from build123d import *

# Parameters (mm, degrees)
CUT_EXTRUDE1_DEPTH      = 18.194103655
CUT_EXTRUDE1_DEPTH_BACK = 18.194103655
SKETCH3_W               = 1
SKETCH3_H               = 11


with BuildPart() as part:
    # Sketch1 → Revolve1 (revolve)
    with BuildSketch(Plane.XY, mode=Mode.PRIVATE) as revolve1_sk:
        Polygon((0, -7), (0, 0), (2.3495, 0), (2.3495, -1.27), (1.7, -1.27), (1.7, -2.92), (1.397, -2.92), (1.397, -14.77), (1.8415, -14.77), (0.889, -16.87), (0.635, -16.87), (0.635, -7), align=None)
    revolve(revolve1_sk.sketch.rotate(Axis((0, -7, 0), (0, 1, 0)), 90), axis=Axis((0, -7, 0), (0, 1, 0)))

    # Sketch3 → Cut-Extrude1 (cut, two sides: drawn at the far end of the back side and taken through both)
    with BuildSketch(Plane.XY.offset(-CUT_EXTRUDE1_DEPTH_BACK)):
        with Locations((0.029190269, -11.37)):
            Rectangle(SKETCH3_W, SKETCH3_H)
    extrude(amount=CUT_EXTRUDE1_DEPTH + CUT_EXTRUDE1_DEPTH_BACK, mode=Mode.SUBTRACT)


solid = part.part
Source: CAD feature listing. Evaluate the final solid. Frame: model axes, mm. A direction names the side the tool comes from. Coordinates: 2 decimals unless noted, no trailing zeros. Loops run counter-clockwise (first coordinate to the right, second up) from the corner with the lowest first, then second, coordinate; pieces in that order, holes last. Notation, with made-up numbers: (78.5, -18.75) -> (129.5, -18.75) arc R20 cw to (129.5, -7.75) -> close; hole circle Ø1 at (11, 79.5). An arc over 180 degrees is marked (long way). Answer in a Markdown table with one row per item. Add a question column.
Q1. Ray query, line 1 along X through (y, z) = (-10, -0.85); line 2 along X through (y, z) = (-11.25, 1.05); line 3 along Y through (x, z) = (1.5, 0.2). Return the intervals inside material, ascending.
Q2. Pull-direction query (X, two-part tool) for faces 1 (the face through (1.24, -8.93, -0.64)), 2 (the face through (0, -5.87, 0)), 3 (the face through (-1.36, -15.83, -0.02)), 4 (the face through (-0.471, -11, 1)); classes: pulls with the +X half, pulls with the -X half, needs draft (parallel to the pull), parting line crosses it, or undercut.
Q3. Reachability of faces 5 (the face through (0.529, -11, 1)), 6 (the face through (-2, -1.27, 0)), 7 (the face through (-1.6, -14.77, 0)) from +Z, -Z, +X, -X, +Y, -Y: full face, straight path, thin tool, end or side. Return the list, or none.
Q4. Section C-C on y = -13. Return the cut outline in (x, z) (3 decimals), and give its area (3 significant figures).
Q5. Section A-A on x = 0. Return the cut outline in (y, z).
Q6. Contact query for flat-ended pins moving along their axis: pin 1 Ø0.7 at (x, z) = (1.5, 0.5) entering from +Y; pin 2 Ø0.8 at (x, z) = (0, -0.5) entering from -Y; pin 3 Ø2 at (y, z) = (-6, 0.5) entering from +X; pin 4 Ø1.1 at (y, z) = (-11, 1) entering from +X. Output: stop coordinate, or through.
Q7. Section D-D on y = -2.5. Return the cut outline in (x, z).
Computed values:
| question | item | result |
|---|---|---|
| 1 | line 1 | x = -1.11 to -0.47, 0.53 to 1.11 |
| 1 | line 2 | x = -0.92 to -0.47, 0.53 to 0.92 |
| 1 | line 3 | y = -15.49 to -14.77, -2.92 to 0 |
| 2 | face 1 | parting line crosses it |
| 2 | face 2 | undercut |
| 2 | face 3 | pulls with the -X half |
| 2 | face 4 | undercut |
| 3 | face 5 | +Z, -Z, -Y |
| 3 | face 6 | none |
| 3 | face 7 | -X |
| 4 | outline | (-0.471, -1.315) -> (-0.471, -0.426) arc R0.635 cw to (-0.471, 0.426) -> (-0.471, 1.315) arc R1.397 ccw to start; (0.529, -1.293) arc R1.397 ccw to (0.529, 1.293) -> (0.529, 0.351) arc R0.635 cw to (0.529, -0.351) -> close |
| 4 | area | 3.25 mm^2 |
| 5 | outline | (-5.87, -1.4) -> (-2.92, -1.4) -> (-2.92, -1.7) -> (-1.27, -1.7) -> (-1.27, -2.35) -> (0, -2.35) -> (0, 2.35) -> (-1.27, 2.35) -> (-1.27, 1.7) -> (-2.92, 1.7) -> (-2.92, 1.4) -> (-5.87, 1.4) -> close |
| 6 | pin 1 | stops at y = 0 |
| 6 | pin 2 | stops at y = -5.87 |
| 6 | pin 3 | stops at x = 1.4 |
| 6 | pin 4 | stops at x = 1.32 |
| 7 | outline | circle Ø3.4 at (0, 0) |
